Source: CAD feature listing. Evaluate the final solid. Frame: model axes, mm. A direction names the side the tool comes from. Give positions to 0.01 mm unless a question says otherwise; leave off trailing zeros. Order: outer loops, then holes, each group sorted by start corner. A loop starts at its lowest first (then second) coordinate and runs counter-clockwise, first axis right, second up. Notation, with made-up numbers: (79.25, 27.5) -> (138.25, 27.5) arc R20 ccw to (138.25, 63.5) -> close; hole circle Ø4 at (3.5, 40.5). An arc over 180 degrees is marked (long way). Use CSV: the item, a comma, the result in double quotes.
```python
from build123d import *

# Parameters (mm, degrees)
BOSS_EXTRUDE1_DEPTH = 5
BOSS_EXTRUDE2_DEPTH = 5
SKETCH3_R           = 49.671400597
CUT_EXTRUDE1_DEPTH  = 3


# Read off the part's stored shape, not the designer's step: Boss-Extrude2
with BuildPart() as part:
    # Sketch1 → Boss-Extrude1 (new body)
    with BuildSketch(Plane.XY):
        with BuildLine():
            Line((-140.302659687, 8.355782272), (-68.12, 8.355782272))
            ThreePointArc((-68.12, 8.355782272), (-64.584466094, 6.891316178), (-63.12, 3.355782272))
            Line((-63.12, 3.355782272), (-63.12, -1.644217728))
            ThreePointArc((-63.12, -1.644217728), (-61.655533906, -5.179751634), (-58.12, -6.644217728))
            Line((-58.12, -6.644217728), (8.507075949, -6.644217728))
            ThreePointArc((8.507075949, -6.644217728), (12.042609855, -5.179751634), (13.507075949, -1.644217728))
            Line((13.507075949, -1.644217728), (13.507075949, 62.750348787))
            ThreePointArc((13.507075949, 62.750348787), (12.042609855, 66.285882693), (8.507075949, 67.750348787))
            Line((8.507075949, 67.750348787), (-42.74804895, 67.750348787))
            ThreePointArc((-42.74804895, 67.750348787), (-46.283582856, 69.214814881), (-47.74804895, 72.750348787))
            Line((-47.74804895, 72.750348787), (-47.74804895, 91.776437317))
            ThreePointArc((-47.74804895, 91.776437317), (-49.212515044, 95.311971223), (-52.74804895, 96.776437317))
            Line((-52.74804895, 96.776437317), (-140.302659687, 96.776437317))
            ThreePointArc((-140.302659687, 96.776437317), (-143.838193593, 95.311971223), (-145.302659687, 91.776437317))
            Line((-145.302659687, 91.776437317), (-145.302659687, 13.355782272))
            ThreePointArc((-145.302659687, 13.355782272), (-143.838193593, 9.820248366), (-140.302659687, 8.355782272))
        make_face()
    extrude(amount=BOSS_EXTRUDE1_DEPTH)

    # Boss-Extrude2 outline → Boss-Extrude2 (add)
    with BuildSketch(Plane(origin=(0, 0, 0), x_dir=(-1, 0, 0), z_dir=(0, 0, -1))):
        Polygon((52.79804895, 91.726437317), (52.79804895, 62.700348787), (-8.457075949, 62.700348787), (-8.457075949, -1.594217728), (58.07, -1.594217728), (58.07, 13.405782272), (140.252659687, 13.405782272), (140.252659687, 91.726437317), align=None)
        Polygon((137.252659687, 16.405782272), (55.79804895, 16.405782272), (55.07, 17.506577949), (55.07, 1.405782272), (-5.457075949, 1.405782272), (-5.457075949, 59.700348787), (55.79804895, 59.700348787), (55.79804895, 88.726437317), (137.252659687, 88.726437317), align=None, mode=Mode.SUBTRACT)
    extrude(amount=BOSS_EXTRUDE2_DEPTH)

    # Sketch3 → Cut-Extrude1 (cut)
    with BuildSketch(Plane.XZ.offset(-88.726437317)):
        with Locations((-95.146165884, -48.5)):
            Circle(SKETCH3_R)
    extrude(amount=-CUT_EXTRUDE1_DEPTH, mode=Mode.SUBTRACT)


solid = part.part
```
1. Ray query, line 1 along Y through (x, z) = (-77.5, -1.25); line 2 along X through (y, z) = (80, -4.25); line 3 along X through (y, z) = (46.5, -0.75). Return the intervals inside material, ascending.
Answer below:
line 1,"y = 13.41 to 16.41, 88.73 to 91.73"
line 2,"x = -140.25 to -137.25, -55.8 to -52.8"
line 3,"x = -140.25 to -137.25, 5.46 to 8.46"
2. Section query A-A on x = -135. Return loops of the section in (y, z).
Answer below:
outline,"(8.36, 0) -> (13.41, 0) -> (13.41, -5) -> (16.41, -5) -> (16.41, 0) -> (88.73, 0) -> (88.73, -5) -> (91.73, -5) -> (91.73, 0) -> (96.78, 0) -> (96.78, 5) -> (8.36, 5) -> close"
3. Section query B-B on y = 54.5. Return loops of the section in (x, z).
Answer below:
outline,"(-145.3, 0) -> (-140.25, 0) -> (-140.25, -5) -> (-137.25, -5) -> (-137.25, 0) -> (5.46, 0) -> (5.46, -5) -> (8.46, -5) -> (8.46, 0) -> (13.51, 0) -> (13.51, 5) -> (-145.3, 5) -> close"
4. Access query for faces 5 (the flat face through (-23, 62.7, -2)), 6 (the flat face through (-105, 8.356, 2)), 7 (the flat face through (-125, 88.726, -2)). Directions: +Z, -Z, +X, -X, +Y, -Y. A direction counts if a zero-diameter tool reaches every point of the face in a straight line with its end or side. Return the directions, or none.
Answer below:
face 5,"-Z, +X, +Y"
face 6,"+Z, -Z, -X, -Y"
face 7,"-Z"
5. Mould query, pull axis X, two halves, no side actions, for faces 1 (the flat face through (8.457, 31, -2)), 2 (the flat face through (-127, 91.726, -2)), 3 (the flat face through (5.457, 30, -2)), 4 (the flat face through (-67, 88.726, -2)). Classes: released by +X, released by -X, zero draft, split by the parting line, or undercut.
Answer below:
face 1,"released by +X"
face 2,"zero draft"
face 3,"undercut"
face 4,"undercut"
6. Pin query (flat end, axial travel): P1, Ø8, axis at x = -101.5, y = 53.5, coming from the -Z side; P2, Ø2.5, axis at x = -39.5, z = -3, coming from the +Y side; P3, Ø4, axis at x = -81.5, z = -2.5, coming from the -Y side. Return the tip coordinate at first contact, or that it passes through.
Answer below:
P1,"stops at z = 0"
P2,"stops at y = 62.7"
P3,"stops at y = 13.41"
7. Section query C-C on z = -3. Return loops of the section in (x, y).
Answer below:
outline,"(-140.25, 13.41) -> (-58.07, 13.41) -> (-58.07, -1.59) -> (8.46, -1.59) -> (8.46, 62.7) -> (-52.8, 62.7) -> (-52.8, 91.73) -> (-75.22, 91.73) -> (-75.22, 88.73) -> (-55.8, 88.73) -> (-55.8, 59.7) -> (5.46, 59.7) -> (5.46, 1.41) -> (-55.07, 1.41) -> (-55.07, 17.51) -> (-55.8, 16.41) -> (-137.25, 16.41) -> (-137.25, 88.73) -> (-115.07, 88.73) -> (-115.07, 91.73) -> (-140.25, 91.73) -> close"
